Work out the finished part from the listing and answer in its coordinate system (mm). Coordinates: 2 decimals unless noted, no trailing zeros. Order: outer loops, then holes, each group sorted by start corner. A loop starts at its lowest first (then second) coordinate and runs counter-clockwise, first axis right, second up. Notation, with made-up numbers: M -22,13.5 L 17,13.5 A22 ccw 17,52.5 Z; hole C 51,-26.5 d1. An arc over 180 degrees is marked long. Use a Markdown table: item, result.
from build123d import *

# Parameters (mm, degrees)
SKETCH_1_W      = 30
SKETCH_1_H      = 15
SKETCH_1_R      = 2
EXTRUDE_1_DEPTH = 5.8
FILLET_1_R      = 3


with BuildPart() as part:
    # ｽｹｯﾁ1 → ﾎﾞｽ - 押し出し1 (new body)
    with BuildSketch(Plane(origin=(0, 0, 0), x_dir=(0, 0, -1), z_dir=(1, 0, 0))):
        Rectangle(SKETCH_1_W, SKETCH_1_H)
        with Locations((10, 0)):
            Circle(SKETCH_1_R, mode=Mode.SUBTRACT)
        with Locations(Location((-10, 0, 0), (0, 0, 180))):
            Circle(SKETCH_1_R, mode=Mode.SUBTRACT)
    extrude(amount=EXTRUDE_1_DEPTH)

    # ﾌｨﾚｯﾄ1
    fillet_1_edges = [part.edges().sort_by_distance(p)[0] for p in [
        (2.9, -7.5, -15),
        (2.9, -7.5, 15),
        (2.9, 7.5, 15),
        (2.9, 7.5, -15),
    ]]
    fillet(fillet_1_edges, radius=FILLET_1_R)


solid = part.part
(1) Determine the mould class of faces 1 (the cylindrical face through (2.9, -1.2, -8.4)), 2 (the flat face through (0, 0, 0)), 3 (the flat face through (3, -7.5, 0)), 4 (the flat face through (3, 7.5, 0)) for opening direction Y: pulls with the +Y half, pulls with the -Y half, needs draft (parallel to the pull), parting line crosses it, or undercut.
Conclusion:
| item | result |
|---|---|
| face 1 | undercut |
| face 2 | needs draft |
| face 3 | pulls with the -Y half |
| face 4 | pulls with the +Y half |
(2) Straight lines are drawn through the part: L1, parallel to Z at x = 1.8, y = -1.25; L2, parallel to Y at x = 3.2, z = -10; L3, parallel to Z at x = 0.3, y = 1.5. For each, find the intervals that lie inside material, in ascending order.
Conclusion:
| item | result |
|---|---|
| L1 | -15 to -11.56, -8.44 to 8.44, 11.56 to 15 |
| L2 | -7.5 to -2, 2 to 7.5 |
| L3 | -15 to -11.32, -8.68 to 8.68, 11.32 to 15 |
(3) A cutting plane is placed at B-B (z = -10). Determine the outline of the cut face in (x, y).
Conclusion:
| item | result |
|---|---|
| outline | M 0,-7.5 L 5.8,-7.5 L 5.8,-2 L 0,-2 Z; M 0,2 L 5.8,2 L 5.8,7.5 L 0,7.5 Z |
(4) A cutting plane is placed at A-A (y = 0). Determine the outline of the cut face in (x, z), then the cut area to 3 significant figures.
Conclusion:
| item | result |
|---|---|
| outline | M 0,-15 L 5.8,-15 L 5.8,-12 L 0,-12 Z; M 0,-8 L 5.8,-8 L 5.8,8 L 0,8 Z; M 0,12 L 5.8,12 L 5.8,15 L 0,15 Z |
| area | 128 mm2 |
(5) A cutting plane is placed at C-C (x = 4.1). Determine the outline of the cut face in (y, z), then the cut area to 3 significant figures.
Conclusion:
| item | result |
|---|---|
| outline | M -7.5,-12 A3 ccw -4.5,-15 L 4.5,-15 A3 ccw 7.5,-12 L 7.5,12 A3 ccw 4.5,15 L -4.5,15 A3 ccw -7.5,12 Z; hole C 0,-10 d4; hole C 0,10 d4 |
| area | 417 mm2 |
(6) A cutting plane is placed at D-D (y = -6.5). Determine the outline of the cut face in (x, z).
Conclusion:
| item | result |
|---|---|
| outline | M 0,-14.24 L 5.8,-14.24 L 5.8,14.24 L 0,14.24 Z |
